Here's how the part is built. I have some questions about the finished solid (model axes, mm). A direction names the side the tool comes from. Round coordinates to 2 decimals unless told otherwise and drop trailing zeros. Write each loop counter-clockwise with the first axis right and the second up, starting at its lowest first coordinate (ties: lowest second). Pieces come first, ordered by that corner, then holes. Notation, with made-up numbers: (16.25, -36) -> (59.25, -36) arc R17 cw to (59.25, -9) -> close; hole circle Ø2 at (-6, 19). An arc over 180 degrees is marked (long way). Put each result on its own line as item: value. Start each with the question number.
1. Suppose I cut it at B-B (z = 26.5). Please give me the cut outline in (x, y), then the cut area to 3 significant figures.
2. Which directions (+Z, -Z, +X, -X, +Y, -Y) give clear straight access to the entire face, cutting with the end or side of a thin tool? Please do faces 1 (the face through (-44.7, 5, 15)), 2 (the face through (46.7, 5, 0)), 3 (the face through (-0.33, 7.48, 25.03)), 4 (the face through (45.714, 3.43, -11.613)), 5 (the face through (-46.7, 5, 0)).
3. I need wall thicknesses on probe 1 along X at (y, z) = (5.25, 20); probe 2 along Y at (x, z) = (0, 23.25); probe 3 along Y at (x, z) = (-45.8, -15.4). Which ranges of each line are inside material? Lowest first, please. Write a range as from..to.
4. Suppose I cut it at A-A (z = 13.05). Please give me the cut outline in (x, y), then the cut area to 3 significant figures.
5. For pin 1 (4 mm diameter, centred on y = 5, z = 14, fed in from +X); pin 2 (2.5 mm diameter, centred on y = 6.5, z = 14, fed in from -X), each with a flat end and sliding along its axis, tell me the tip position at first contact or that it passes through.
6. Suppose I cut it at C-C (y = 5). Please give me the cut outline in (x, z), then the cut area to 3 significant figures.
7. We'd pull the mould along Z, two halves only. Please class faces 6 (the face through (44.7, 5, 15)), 7 (the face through (-1, 2, 30.8)), 8 (the face through (-45.714, 6.57, 11.613)), 9 (the face through (-1, 10, 0)): +Z half, -Z half, draft (parallel to the pull), parting line (faces both ways), or undercut.
```python
from build123d import *

# Parameters (mm, degrees)
CROQUIS1_W                 = 93.4
CROQUIS1_H                 = 61.6
CROQUIS1_R                 = 6.55
SALIENTE_EXTRUIR1_DEPTH    = 10
CROQUIS2_R                 = 4.1
CORTAR_EXTRUIR1_DEPTH      = 2
CORTAR_EXTRUIR2_REACH      = 79.945
CORTAR_EXTRUIR2_END_RADIUS = 6.55
CROQUIS3_R                 = 2.5


with BuildPart() as part:
    # Croquis1 → Saliente-Extruir1 (new body)
    with BuildSketch(Plane(origin=(0, 0, 0), x_dir=(1, 0, 0), z_dir=(0, 1, 0))):
        Rectangle(CROQUIS1_W, CROQUIS1_H)
        with Locations(Location((0, -13.05, 0), (0, 0, 270))):
            Circle(CROQUIS1_R, mode=Mode.SUBTRACT)
    extrude(amount=SALIENTE_EXTRUIR1_DEPTH)

    # Croquis2 → Cortar-Extruir1 (cut)
    with BuildSketch(Plane.ZY.offset(46.7)):
        with Locations((-15.4, 5)):
            Circle(CROQUIS2_R)
        with Locations(Location((15.4, 5, 0), (0, 0, 180))):
            Circle(CROQUIS2_R)
    cortar_extruir1 = extrude(amount=-CORTAR_EXTRUIR1_DEPTH, mode=Mode.SUBTRACT)

    # Simetría2: Cortar-Extruir1 across plane
    add(cortar_extruir1.mirror(Plane(origin=(0, 0, 0), x_dir=(0, 0, 1), z_dir=(1, 0, 0))), mode=Mode.SUBTRACT)

    # Cortar-Extruir2: up to this cylinder (the profile starts outside it)
    cortar_extruir2_end = Plane(origin=(0, 5, 13.05), z_dir=(0, -1, 0)) * Cylinder(CORTAR_EXTRUIR2_END_RADIUS, 173.99, mode=Mode.PRIVATE)
    # Croquis3 → Cortar-Extruir2 (cut, up to the surface)
    with BuildSketch(Plane.XY.offset(30.8), mode=Mode.PRIVATE) as cortar_extruir2_sk1:
        with Locations((0, 5)):
            Circle(CROQUIS3_R)
    cortar_extruir2_tool1 = extrude(cortar_extruir2_sk1.sketch, amount=-CORTAR_EXTRUIR2_REACH, mode=Mode.PRIVATE) - cortar_extruir2_end
    add(cortar_extruir2_tool1.solids().sort_by_distance((0, 5, 30.8))[0], mode=Mode.SUBTRACT)


solid = part.part
```
Verdict:
1. outline: (-46.7, 0) -> (46.7, 0) -> (46.7, 10) -> (-46.7, 10) -> close; hole circle Ø5 at (0, 5)
1. area: 914 mm^2
2. face 1: -X
2. face 2: +Z, -Z, +X, +Y, -Y
2. face 3: +Z
2. face 4: +X
2. face 5: +Z, -Z, -X, +Y, -Y
3. probe 1: x = -46.7..-2.49, 2.49..46.7
3. probe 2: y = 0..2.5, 7.5..10
3. probe 3: y = 0..0.9, 9.1..10
4. outline: (-46.7, 0) -> (-6.55, 0) -> (-6.55, 10) -> (-46.7, 10) -> (-46.7, 8.36) -> (-44.7, 8.36) -> (-44.7, 1.64) -> (-46.7, 1.64) -> close; (6.55, 0) -> (46.7, 0) -> (46.7, 1.64) -> (44.7, 1.64) -> (44.7, 8.36) -> (46.7, 8.36) -> (46.7, 10) -> (6.55, 10) -> close
4. area: 776 mm^2
5. pin 1: stops at x = 44.7
5. pin 2: stops at x = -44.7
6. outline: (-46.7, -30.8) -> (46.7, -30.8) -> (46.7, -19.5) -> (44.7, -19.5) -> (44.7, -11.3) -> (46.7, -11.3) -> (46.7, 11.3) -> (44.7, 11.3) -> (44.7, 19.5) -> (46.7, 19.5) -> (46.7, 30.8) -> (2.5, 30.8) -> (2.5, 19.1) arc R6.55 cw (long way) to (-2.5, 19.1) -> (-2.5, 30.8) -> (-46.7, 30.8) -> (-46.7, 19.5) -> (-44.7, 19.5) -> (-44.7, 11.3) -> (-46.7, 11.3) -> (-46.7, -11.3) -> (-44.7, -11.3) -> (-44.7, -19.5) -> (-46.7, -19.5) -> close
6. area: 5,500 mm^2
7. face 6: undercut
7. face 7: +Z half
7. face 8: undercut
7. face 9: draft
